Input: part model. Units: mm. Frame: model coordinates. A direction names the side the tool comes from. Give positions to 0.01 mm unless a question says otherwise; leave off trailing zeros. Loops run counter-clockwise (first coordinate to the right, second up) from the corner with the lowest first, then second, coordinate; pieces in that order, holes last. Notation, with made-up numbers: M 11,19.5 L 41,19.5 A32 cw 41,49.5 Z; hole C 31,32.5 d9. An arc over 180 degrees is marked long. Use CSV: the item, a comma, the result in double quotes. Start each with the question number.
Q1. Material intervals for line 1 along X through (y, z) = (-8.2, 7.5) (3 decimals); line 2 along Y through (x, z) = (3.75, 6.25); line 3 along X through (y, z) = (-7, 16.5) (3 decimals), sorted ascending.
Q2. Section D-D, the plane x = 2. Output: boundary loops of the cut face in (y, z), plus the area to 3 significant figures.
Q3. Section A-A, the plane y = -9.5. Output: boundary loops of the cut face in (x, z).
Q4. Pin query (flat end, axial travel): pin 1 (5 mm diameter, centred on x = 18.5, y = 0, fed in from +Z); pin 2 (8 mm diameter, centred on y = -18, z = 15.5, fed in from +X); pin 3 (1.5 mm diameter, centred on x = 15, z = 13.5, fed in from -Y); pin 4 (5 mm diameter, centred on y = 0.5, z = 5, fed in from +X). Return the tip coordinate at first contact, or that it passes through.
Q5. Section C-C, the plane z = 11.5. Output: boundary loops of the cut face in (x, y).
Q6. Reachability of faces 4 (the flat face through (9, 6, 3)), 5 (the flat face through (3, -19.4, 6.2)), 6 (the flat face through (19.42, -9, 6.27)) from +Z, -Z, +X, -X, +Y, -Y: full face, straight path, thin tool, end or side. Return the list, or none.
Q7. Pull-direction query (X, two-part tool) for faces 1 (the flat face through (20.48, -10.521, 6.095)), 2 (the cylindrical face through (0.43, -6.25, 0.45)), 3 (the cylindrical face through (11.55, -17.34, 0.43)); classes: released by +X, released by -X, zero draft, split by the parting line, or undercut.
Q8. Section B-B, the plane x = 18. Output: boundary loops of the cut face in (y, z) (3 decimals).
Autodesk Inventor part; units mm, degrees
ref_plane "YZ Plane" through (0, 0, 0) normal (1, 0, 0) x (0, 1, 0)
ref_plane "XZ Plane" through (0, 0, 0) normal (0, 1, 0) x (-1, 0, 0)
ref_plane "XY Plane" through (0, 0, 0) normal (0, 0, 1) x (1, 0, 0)
sketch "Sketch1" plane through (0, 0, 0) normal (0, 0, 1) x (1, 0, 0)
  line L0 (0, 0) -> (12, 0)
  line L1 (12, 0) -> (12, 12)
  line L2 (12, 12) -> (0, 12)
  line L3 (0, 12) -> (0, 0)
  line L4 (12, 0) -> (0, 0)
  line L5 (0, 0) -> (0, -12)
  line L6 (0, -12) -> (12, -12)
  line L7 (12, -12) -> (12, 0)
  line L8 (12, 0) -> (24, 0)
  line L9 (24, 0) -> (24, -12)
  line L10 (24, -12) -> (12, -12)
  line L11 (12, -12) -> (12, 0)
  line L12 (0, -12) -> (-12, -12)
  line L13 (-12, -12) -> (-12, 0)
  line L14 (-12, 0) -> (0, 0)
  line L15 (0, 0) -> (0, -12)
  line L16 (0, -12) -> (12, -12)
  line L17 (12, -12) -> (12, -24)
  line L18 (12, -24) -> (0, -24)
  line L19 (0, -24) -> (0, -12)
  dimension "d0" = 12
  dimension "d1" = 12
  dimension "d2" = 12
  dimension "d3" = 12
  dimension "d4" = 12
  dimension "d5" = 12
  dimension "d6" = 12
  dimension "d7" = 12
  dimension "d8" = 12
  dimension "d9" = 12
extrude "Extrusion1" add sketch "Sketch1" along normal blind 3
sketch "Sketch2" plane through (0, 0, 3) normal (0, 0, 1) x (1, 0, 0)
  line L0 (-12, 0) -> (-12, -12)
  line L1 (-12, -12) -> (-12, -6)
  line L2 (-12, -6) -> (0, -6)
  line L3 (-12, -12) -> (0, -12)
  line L4 (0, -6) -> (0, -12)
  line L5 (0, -12) -> (-12, -12)
  line L6 (12, -24) -> (12, -12)
  line L7 (12, -12) -> (12, -6)
  line L8 (12, -6) -> (24, -6)
  line L9 (24, -12) -> (24, 0)
  line L10 (12, -12) -> (24, -12)
  line L11 (24, -6) -> (24, -12)
  line L12 (24, -12) -> (12, -12)
  line L13 (0, 0) -> (0, -6)
  line L14 (12, 0) -> (12, 12)
  line L15 (0, 0) -> (12, 0)
  line L16 (12, 0) -> (12, -6)
  line L17 (12, -12) -> (0, -12)
  line L18 (0, 12) -> (0, 0)
  line L19 (0, 0) -> (0, 12)
  line L20 (0, 12) -> (6, 12)
  line L21 (12, 12) -> (0, 12)
  line L22 (6, 12) -> (6, 0)
  line L23 (6, 0) -> (0, 0)
  line L24 (0, -12) -> (0, -24)
  line L25 (0, -12) -> (0, -24)
  line L26 (0, -24) -> (6, -24)
  line L27 (0, -24) -> (12, -24)
  line L28 (6, -24) -> (6, -12)
  line L29 (6, -12) -> (0, -12)
  dimension "d12" = 6
  dimension "d13" = 12
extrude "Extrusion2" add sketch "Sketch2" along normal blind 9 contours L2 L4 L3 L0 | L13 L15 L16 L7 L17 L4 | L17 L28 L26 L24 | L18 L20 L22 L15 | L7 L8 L9 L10
sketch "Sketch3" plane through (0, 0, 12) normal (0, 0, 1) x (1, 0, 0)
  line L0 (0, -6) -> (12, -6)
  line L1 (12, -12) -> (6, -12)
  line L2 (12, -6) -> (12, -12)
  line L3 (0, -12) -> (0, -24)
  line L4 (12, -12) -> (0, -12)
  line L5 (0, -12) -> (0, -6)
  point P0 (0, 0)
extrude "Extrusion3" add sketch "Sketch3" along normal blind 9
sketch "Sketch4" plane through (6, -12, 3) normal (0, -1, 0) x (1, 0, 0)
  point P0 (-6, -3)
sketch "Sketch5" plane through (-12, -6, 3) normal (0, 1, 0) x (1, 0, 0)
  circle A0 centre (6, -4.5) radius 1.725
  line L0 (0, 0) -> (0, -9)
  line L1 (12, -9) -> (0, -9)
  circle A1 centre (18, -13.5) radius 1.725
  line L2 (24, -18) -> (12, -18)
  line L3 (24, -9) -> (24, -18)
  circle A2 centre (30, -4.5) radius 1.725
  line L4 (36, 0) -> (36, -9)
  line L5 (36, -9) -> (24, -9)
  point P0 (12, 3)
  dimension "d19" = 3.45
  dimension "d20" = 6
  dimension "d21" = 4.5
  dimension "d22" = 3.45
  dimension "d23" = 4.5
  dimension "d24" = 6
  dimension "d25" = 3.45
  dimension "d26" = 6
  dimension "d27" = 4.5
extrude "Extrusion4" cut sketch "Sketch5" against normal blind 3
sketch "Sketch6" plane through (6, -12, 3) normal (0, -1, 0) x (1, 0, 0)
  circle A0 centre (-12, 4.5) radius 1.725
  line L0 (-10.3546, 7.35) -> (-8.7091, 4.5)
  line L1 (-8.7091, 4.5) -> (-10.3546, 1.65)
  line L2 (-10.3546, 1.65) -> (-13.6454, 1.65)
  line L3 (-13.6454, 1.65) -> (-15.2909, 4.5)
  line L4 (-15.2909, 4.5) -> (-13.6454, 7.35)
  line L5 (-13.6454, 7.35) -> (-10.3546, 7.35)
  circle A1 centre (12, 4.5) radius 1.725
  line L6 (13.6454, 7.35) -> (15.2909, 4.5)
  line L7 (15.2909, 4.5) -> (13.6454, 1.65)
  line L8 (13.6454, 1.65) -> (10.3546, 1.65)
  line L9 (10.3546, 1.65) -> (8.7091, 4.5)
  line L10 (8.7091, 4.5) -> (10.3546, 7.35)
  line L11 (10.3546, 7.35) -> (13.6454, 7.35)
  circle A2 centre (0, 13.5) radius 1.725
  line L12 (1.6454, 16.35) -> (3.2909, 13.5)
  line L13 (3.2909, 13.5) -> (1.6454, 10.65)
  line L14 (1.6454, 10.65) -> (-1.6454, 10.65)
  line L15 (-1.6454, 10.65) -> (-3.2909, 13.5)
  line L16 (-3.2909, 13.5) -> (-1.6454, 16.35)
  line L17 (-1.6454, 16.35) -> (1.6454, 16.35)
  point P0 (-6, -3)
  dimension "d30" = 2.85
  dimension "d31" = 2.85
  dimension "d32" = 2.85
extrude "Extrusion5" cut sketch "Sketch6" against normal blind 3 contours A0 | L0 L1 L2 L3 L4 L5 | A1 | L6 L7 L8 L9 L10 L11 | A2 | L12 L13 L14 L15 L16 L17
sketch "Sketch7" plane through (6, 0, 3) normal (1, 0, 0) x (0, 0, -1)
  circle A0 centre (-4.5, 6) radius 1.725
  circle A1 centre (-4.5, -18) radius 1.725
  line L0 (-9, 0) -> (-9, 12)
  line L1 (-9, -24) -> (-9, -12)
  line L2 (0, -24) -> (-9, -24)
  line L3 (0, 12) -> (-9, 12)
  point P0 (3, 0)
  dimension "d35" = 3.45
  dimension "d36" = 3.45
  dimension "d37" = 4.5
  dimension "d38" = 4.5
  dimension "d39" = 6
  dimension "d40" = 6
extrude "Extrusion6" cut sketch "Sketch7" against normal blind 3
sketch "Sketch8" plane through (0, -6, 3) normal (-1, 0, 0) x (0, 0, 1)
  circle A0 centre (4.5, 12) radius 1.725
  line L0 (1.65, 13.6454) -> (4.5, 15.2909)
  line L1 (4.5, 15.2909) -> (7.35, 13.6454)
  line L2 (7.35, 13.6454) -> (7.35, 10.3546)
  line L3 (7.35, 10.3546) -> (4.5, 8.7091)
  line L4 (4.5, 8.7091) -> (1.65, 10.3546)
  line L5 (1.65, 10.3546) -> (1.65, 13.6454)
  circle A1 centre (4.5, -12) radius 1.725
  line L6 (1.65, -10.3546) -> (4.5, -8.7091)
  line L7 (4.5, -8.7091) -> (7.35, -10.3546)
  line L8 (7.35, -10.3546) -> (7.35, -13.6454)
  line L9 (7.35, -13.6454) -> (4.5, -15.2909)
  line L10 (4.5, -15.2909) -> (1.65, -13.6454)
  line L11 (1.65, -13.6454) -> (1.65, -10.3546)
  point P0 (-3, 6)
  dimension "d43" = 2.85
  dimension "d44" = 2.85
extrude "Extrusion7" cut sketch "Sketch8" against normal blind 3 contours A0 | L0 L1 L2 L3 L4 L5 | A1 | L6 L7 L8 L9 L10 L11
sketch "Sketch9" plane through (0, 0, 0) normal (0, 0, -1) x (-1, 0, 0)
  line L0 (0, 0) -> (12, 0)
  line L1 (12, 0) -> (12, -12)
  line L2 (0, 0) -> (12, 0)
  line L3 (12, 0) -> (12, -12)
  line L4 (12, -12) -> (0, -12)
  line L5 (0, -12) -> (0, 0)
extrude "Extrusion8" cut sketch "Sketch9" against normal through all
fillet "Fillet2" radius 1.5 5 edges at (18, 0, 0) (12, 6, 0) (18, -12, 0) (12, -18, 0) (0, -6, 0)
properties part number "threewayNSW"
A:
1,line 1,"0 to 16.275, 19.725 to 24"
1,line 2,"-24 to -19.19, -16.81 to 4.81, 7.19 to 12"
1,line 3,"0 to 4.275, 7.725 to 12"
2,outline,"M -24,0 L 12,0 L 12,12 L -6,12 L -6,21 L -12,21 L -12,12 L -24,12 Z; hole M -21.29,7.5 L -19.65,4.65 L -16.35,4.65 L -14.71,7.5 L -16.35,10.35 L -19.65,10.35 Z; hole M 2.71,7.5 L 4.35,4.65 L 7.65,4.65 L 9.29,7.5 L 7.65,10.35 L 4.35,10.35 Z"
2,area,"430 mm^2"
3,outline,"M 0,1.5 A1.5 ccw 1.5,0 L 24,0 L 24,12 L 12,12 L 12,21 L 0,21 Z; hole M 2.71,16.5 L 4.35,13.65 L 7.65,13.65 L 9.29,16.5 L 7.65,19.35 L 4.35,19.35 Z; hole M 14.71,7.5 L 16.35,4.65 L 19.65,4.65 L 21.29,7.5 L 19.65,10.35 L 16.35,10.35 Z"
4,pin 1,"z = 3"
4,pin 2,"x = 6"
4,pin 3,"through"
4,pin 4,"x = 24"
5,outline,"M 0,-24 L 6,-24 L 6,-12 L 24,-12 L 24,-6 L 12,-6 L 12,0 L 6,0 L 6,12 L 0,12 Z"
6,face 4,"+Z, +X, +Y"
6,face 5,"-X"
6,face 6,"-Y"
7,face 1,"undercut"
7,face 2,"released by -X"
7,face 3,"released by +X"
8,outline,"M -12,1.5 A1.5 ccw -10.5,0 L -1.5,0 A1.5 ccw 0,1.5 L 0,3 L -6,3 L -6,5.775 L -9,5.775 L -9,4.65 L -12,4.65 Z; M -12,10.35 L -9,10.35 L -9,9.225 L -6,9.225 L -6,12 L -12,12 Z"
